Geometry: see drawing. Coordinates: mm, zero at the bounding-box minimum. A direction names the side the tool comes from. Give positions to 0.01 mm unless a question says otherwise; leave off trailing zeros. Write each loop counter-clockwise with the first axis right and the second up, starting at its lowest first coordinate (ties: lowest second). Pieces come first, ordered by that corner, then holes. Notation, with made-up numbers: (-32.5, 78) -> (17.5, 78) arc R20 ccw to (17.5, 114) -> close; hole circle Ø6 at (60.25, 88). An arc over 180 degrees is marked (long way). Use CSV: the item, a comma, the result in double quotes. Start each with the question number.
1) Material intervals for line 1 (Y direction, x = 9.5, z = 6.75); line 2 (Y direction, x = 9.5, z = 16.5), sorted ascending. Write a range as [from, to].
2) Contact query for flat-ended pins moving along their axis: P1, Ø5, axis at x = 11, y = 9, coming from the -Z side; P2, Ø6, axis at y = 9, z = 10.5, coming from the +X side; P3, Ø1.5, axis at x = 5.5, z = 4, coming from the -Y side; P4, Ø3, axis at x = 6.5, z = 5, coming from the -Y side. Output: stop coordinate, or through.
3) Draft query along X for the marked faces 1 and 2. Return one class per face: pulls with the +X half, pulls with the -X half, needs draft (parallel to the pull), parting line crosses it, or undercut.
4) Section A-A (y = 9.5). Output: boundary loops of the cut face in (x, z), plus the area to 3 significant figures.
5) Set-up query: the marked faces 3 and 4. Return all of +Z, -Z, +X, -X, +Y, -Y with unobstructed straight access to the full face (end or side cutting, diameter ignored); none if empty.
6) Section C-C (z = 2.75). Output: boundary loops of the cut face in (x, y).
7) Section D-D (y = 15). Output: boundary loops of the cut face in (x, z), plus the area to 3 significant figures.
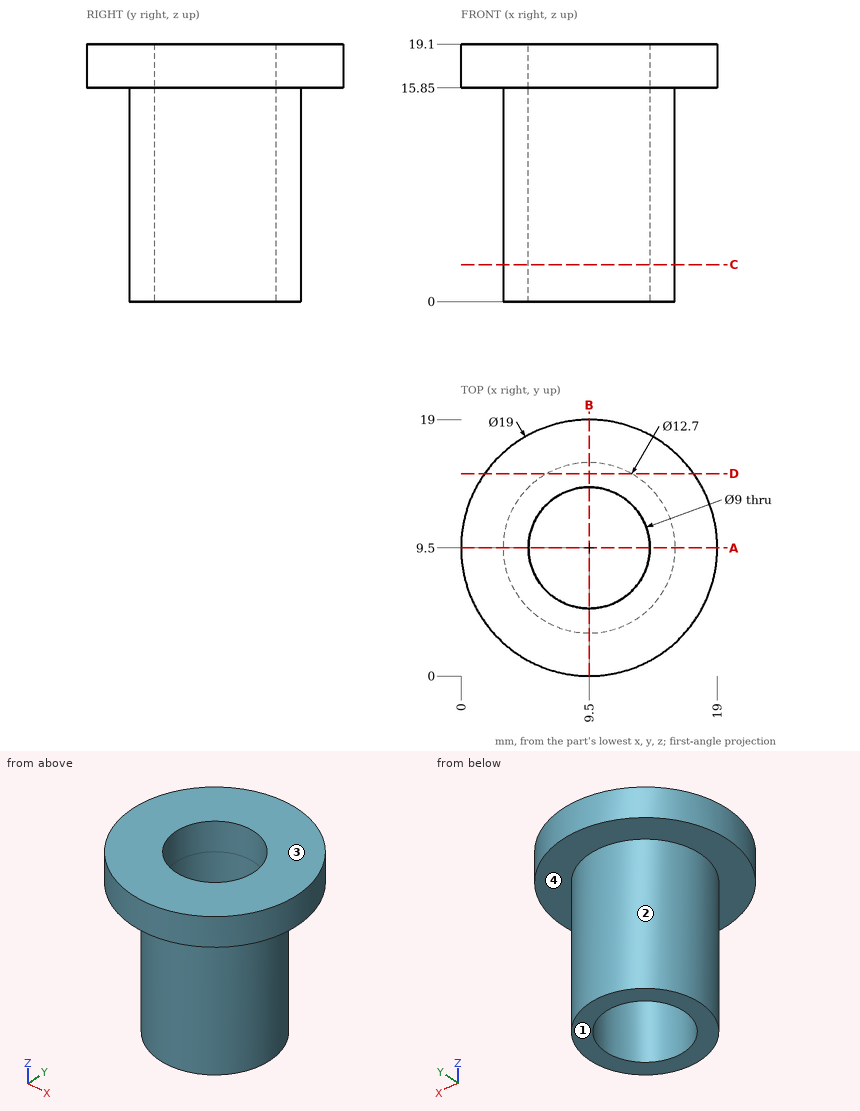
Answers follow:
1,line 1,"y = [3.15, 5], [14, 15.85]"
1,line 2,"y = [0, 5], [14, 19]"
2,P1,"passes through"
2,P2,"stops at x = 15.85"
2,P3,"stops at y = 4.04"
2,P4,"stops at y = 3.33"
3,face 1,"needs draft"
3,face 2,"parting line crosses it"
4,outline,"(0, 15.85) -> (3.15, 15.85) -> (3.15, 0) -> (5, 0) -> (5, 19.1) -> (0, 19.1) -> close; (14, 0) -> (15.85, 0) -> (15.85, 15.85) -> (19, 15.85) -> (19, 19.1) -> (14, 19.1) -> close"
4,area,"91.1 mm^2"
5,face 3,"+Z, +X, -X, +Y, -Y"
5,face 4,"-Z"
6,outline,"circle Ø12.7 at (9.5, 9.5); hole circle Ø9 at (9.5, 9.5)"
7,outline,"(1.75, 15.85) -> (6.33, 15.85) -> (6.33, 0) -> (12.67, 0) -> (12.67, 15.85) -> (17.25, 15.85) -> (17.25, 19.1) -> (1.75, 19.1) -> close"
7,area,"151 mm^2"
